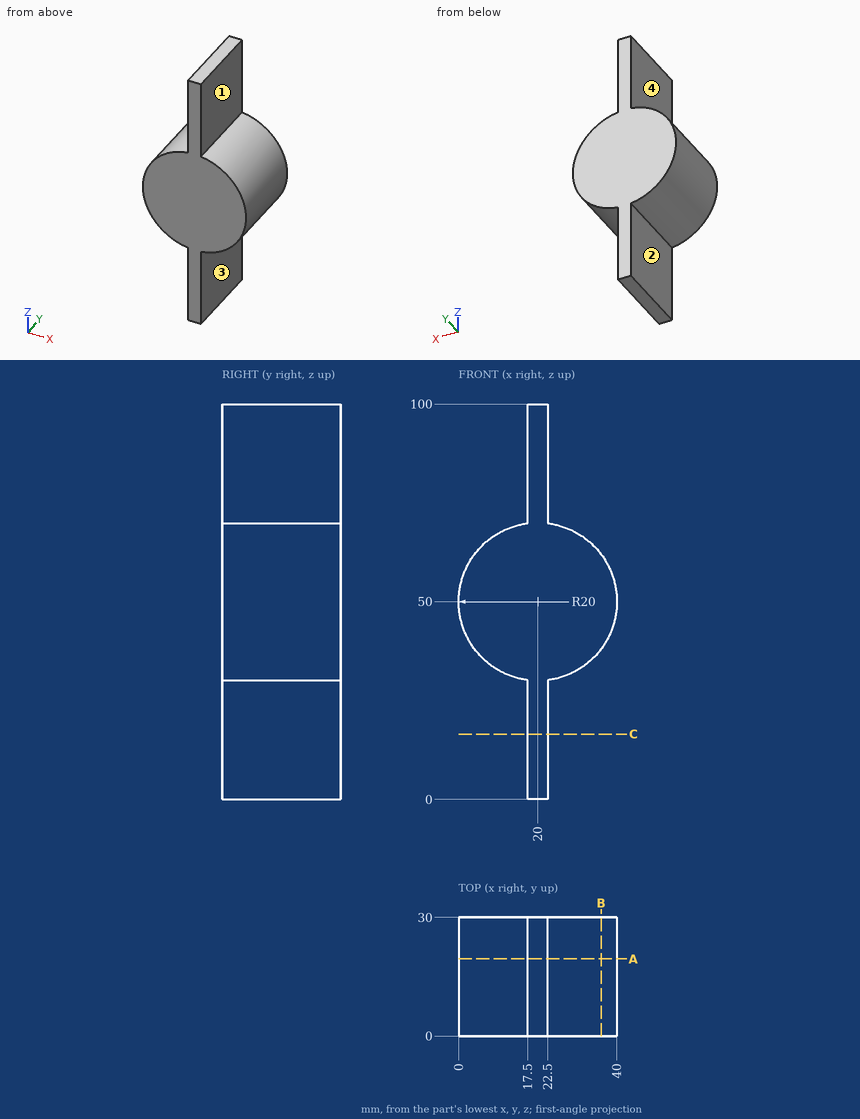
Print and shaded views of the part. All mm, measured from the part's lowest x, y and z. A direction names the side the tool comes from. Round coordinates to 2 decimals unless told otherwise and drop trailing zeros. Write each loop counter-clockwise with the first axis right and the second up, starting at its lowest first coordinate (ties: lowest second). Pieces come first, ordered by that corner, then holes. Notation, with made-up numbers: (-20, 1.25) - (24, 1.25) arc R28 cw to (24, 24.25) - close; hole circle Ø2 at (39, -6). An arc over 180 degrees is marked (long way). Write each question's results on one line, items separated by ' | '. Start each with the question number.
Item 1: Drop flat-ended pins along their axis: P1, Ø1.5, axis at y = 24, z = 31.5, coming from the +X side; P2, Ø8, axis at y = 23.5, z = 72.5, coming from the +X side; P3, Ø10, axis at y = 20, z = 66.5, coming from the -X side. Give the stop position or say it passes through.
Item 2: Saw through at B-B (x = 36). Write the cut outline in (y, z), and give its area (3 significant figures).
Item 3: Saw through at A-A (y = 19.5). Write the cut outline in (x, z), and give its area (3 significant figures).
Item 4: Wall check: L1, parallel to X at y = 16.5, z = 21; L2, parallel to X at y = 14.25, z = 50; L3, parallel to Z at x = 25, y = 20. Give the ranges that are in metal, low to high. Write a range as [from, to].
Item 5: Which spindle directions (+Z, -Z, +X, -X, +Y, -Y) get a long thin tool onto all of the face, cutting with end or side? Do the marked faces 1, 2, 3 and 4. Say none if no direction does.
Item 6: Saw through at C-C (z = 16.5). Write the cut outline in (x, y).
Results are:
1) P1: stops at x = 29.22 | P2: stops at x = 27.6 | P3: stops at x = 3.64
2) outline: (0, 38) - (30, 38) - (30, 62) - (0, 62) - close | area: 720 mm²
3) outline: (17.5, 0) - (22.5, 0) - (22.5, 30.16) arc R20 ccw to (22.5, 69.84) - (22.5, 100) - (17.5, 100) - (17.5, 69.84) arc R20 ccw to (17.5, 30.16) - close | area: 1,560 mm²
4) L1: x = [17.5, 22.5] | L2: x = [0, 40] | L3: z = [30.64, 69.36]
5) face 1: +Z, +X, +Y, -Y | face 2: -Z, -X, +Y, -Y | face 3: -Z, +X, +Y, -Y | face 4: +Z, -X, +Y, -Y
6) outline: (17.5, 0) - (22.5, 0) - (22.5, 30) - (17.5, 30) - close
